For this review, take the finished solid that the model builds, in its own axes (mm). A direction names the side the tool comes from. Coordinates: 2 decimals unless noted, no trailing zeros. Loops run counter-clockwise (first coordinate to the right, second up) from the corner with the lowest first, then second, coordinate; pieces in that order, holes last. Notation, with made-up numbers: M 78.5,-39.75 L 121.5,-39.75 A22 cw 121.5,-12.75 Z; hole C 7,4.5 d7. An arc over 180 degrees is marked long. Put each result on its own line as item: value.
```python
from build123d import *

# Parameters (mm, degrees)
BOSS_EXTRUDE1_DEPTH     = 12
BOSS_EXTRUDE3_DEPTH     = 2
FILLET2_R               = 1
CUT_EXTRUDE7_DEPTH      = 3
CUT_EXTRUDE8_DEPTH      = 1
CUT_EXTRUDE8_DEPTH_BACK = 1


with BuildPart() as part:
    # Sketch1 → Boss-Extrude1 (new body)
    with BuildSketch(Plane.XY):
        with BuildLine():
            Line((3.5, 10), (-3.5, 10))
            ThreePointArc((-3.5, 10), (-5.340169944, 7.795084972), (-6, 5))
            Line((-6, 5), (-6, 0))
            Line((-6, 0), (-7, 0))
            Line((-7, 0), (-7, 1))
            Line((-7, 1), (-7, 5))
            ThreePointArc((-7, 5), (-6.155773268, 8.395374624), (-3.819705149, 11))
            Line((-3.819705149, 11), (3.819705149, 11))
            ThreePointArc((3.819705149, 11), (6.155773268, 8.395374624), (7, 5))
            Line((7, 5), (7, 1))
            Line((7, 1), (7, 0))
            Line((7, 0), (6, 0))
            Line((6, 0), (6, 5))
            ThreePointArc((6, 5), (5.340169944, 7.795084972), (3.5, 10))
        make_face()
    extrude(amount=-BOSS_EXTRUDE1_DEPTH)

    # Sketch4 → Boss-Extrude3 (add)
    with BuildSketch(Plane.XZ):
        with BuildLine():
            Line((-7, 0), (-8.5, 0))
            ThreePointArc((-8.5, 0), (-11.809401077, -3.309401077), (-8.5, -6.618802154))
            Line((-8.5, -6.618802154), (-7, -6.618802154))
            Line((-7, -6.618802154), (-7, 0))
        make_face()
        with BuildLine():
            ThreePointArc((8.5, -6.618802154), (11.809401077, -3.309401077), (8.5, 0))
            Line((8.5, 0), (7, 0))
            Line((7, 0), (7, -6.618802154))
            Line((7, -6.618802154), (8.5, -6.618802154))
        make_face()
    extrude(amount=-BOSS_EXTRUDE3_DEPTH)

    # Fillet2
    fillet2_edges = [part.edges().sort_by_distance(p)[0] for p in [
        (-7, 2, -3.309401077),
        (7, 2, -3.309401077),
    ]]
    fillet(fillet2_edges, radius=FILLET2_R)

    # Sketch5 → Cut-Extrude7 (cut)
    with BuildSketch(Plane(origin=(0, 2, 0), x_dir=(1, 0, 0), z_dir=(0, 1, 0))):
        with BuildLine():
            Line((-7, 4.309401077), (-8, 4.309401077))
            ThreePointArc((-8, 4.309401077), (-9, 3.309401077), (-8, 2.309401077))
            Line((-8, 2.309401077), (-7, 2.309401077))
            Line((-7, 2.309401077), (-3.819705149, 2.309401077))
            Line((-3.819705149, 2.309401077), (-3.819705149, 4.309401077))
            Line((-3.819705149, 4.309401077), (-7, 4.309401077))
        make_face()
        with BuildLine():
            Line((3.819705149, 2.309401077), (7, 2.309401077))
            Line((7, 2.309401077), (8, 2.309401077))
            ThreePointArc((8, 2.309401077), (9, 3.309401077), (8, 4.309401077))
            Line((8, 4.309401077), (7, 4.309401077))
            Line((7, 4.309401077), (3.819705149, 4.309401077))
            Line((3.819705149, 4.309401077), (3.819705149, 2.309401077))
        make_face()
    extrude(amount=-CUT_EXTRUDE7_DEPTH, mode=Mode.SUBTRACT)

    # Sketch6 → Cut-Extrude8 (cut, two sides)
    with BuildSketch(Plane(origin=(0, 2, 0), x_dir=(1, 0, 0), z_dir=(0, 1, 0))) as cut_extrude8_sk:
        Polygon((-8, 5.618802154), (-10, 4.464101615), (-10, 2.154700538), (-8, 1), (-6, 1), (-6, 5.618802154), align=None)
        Polygon((6, 1), (8, 1), (10, 2.154700538), (10, 4.464101615), (8, 5.618802154), (6, 5.618802154), align=None)
    extrude(amount=CUT_EXTRUDE8_DEPTH, mode=Mode.SUBTRACT)
    extrude(cut_extrude8_sk.sketch, amount=-CUT_EXTRUDE8_DEPTH_BACK, mode=Mode.SUBTRACT)


solid = part.part
```
(1) Add section C-C (z = -9). Write out the cut boundary in (x, y).
Determined:
outline: M -7,0 L -6,0 L -6,5 A6.25 cw -3.5,10 L 3.5,10 A6.25 cw 6,5 L 6,0 L 7,0 L 7,5 A7.25 ccw 3.82,11 L -3.82,11 A7.25 ccw -7,5 Z
(2) Add section A-A (y = 4). Write out the cut boundary in (x, z), plus the area to 3 significant figures.
Determined:
outline: M -7,-12 L -6,-12 L -6,0 L -7,0 Z; M 6,-12 L 7,-12 L 7,0 L 6,0 Z
area: 24.0 mm^2
(3) Wall thickness on line 1 along X through (y, z) = (5.25, -4.25) (3 decimals); line 2 along Y through (x, z) = (0.75, -8.25); line 3 along X through (y, z) = (9.25, -9.5): over which ranges is each line inside the solid? List them lowest first. Write a range as [from, to].
Determined:
line 1: x = [-6.996, -5.995], [5.995, 6.996]
line 2: y = [10, 11]
line 3: x = [-5.62, -4.33], [4.33, 5.62]
(4) Add section D-D (y = 1.5). Write out the cut boundary in (x, z), plus the area to 3 significant figures.
Determined:
outline: M -10,-4.46 L -10,-2.15 L -8,-1 L -6,-1 L -6,0 L -8.5,0 A3.31 ccw -8.5,-6.62 L -7,-6.62 L -7,-12 L -6,-12 L -6,-5.62 L -8,-5.62 Z; M 6,-12 L 7,-12 L 7,-6.62 L 8.5,-6.62 A3.31 ccw 8.5,0 L 6,0 L 6,-1 L 8,-1 L 10,-2.15 L 10,-4.46 L 8,-5.62 L 6,-5.62 Z
area: 45.9 mm^2
(5) Draft analysis for pull direction Y (two halves, no side actions). For faces 1 (the flat face through (0, 11, -6)), 2 (the flat face through (6.5, 3, -3.3)), 3 (the flat face through (-9, 1, -4)), 4 (the flat face through (-7, 3, -7)), state which applies: +Y half, -Y half, draft (parallel to the pull), parting line (faces both ways), or undercut.
Determined:
face 1: +Y half
face 2: undercut
face 3: undercut
face 4: draft
(6) Tool access review of faces 5 (the flat face through (-10.4, 2, -3.3)), 6 (the flat face through (7, 2, -1)), 7 (the flat face through (-10, 1.5, -3.3)): name each direction out of +Z, -Z, +X, -X, +Y, -Y from which nothing blocks a thin tool from reaching the whole face with its end or side.
Determined:
face 5: +Z, -Z, -X, +Y
face 6: none
face 7: +Y
(7) For pin 1 (4 mm diameter, centred on y = 3, z = -5.5, fed in from -X); pin 2 (3 mm diameter, centred on x = -10, z = -2, fed in from +Y); pin 3 (1.5 mm diameter, centred on y = 8, z = -9, fed in from +X); pin 4 (2 mm diameter, centred on x = 9.5, z = -10, fed in from -Y), all flat-tipped, find the tip position at first contact; note any pin that passes through.
Determined:
pin 1: stops at x = -11.78
pin 2: stops at y = 2
pin 3: stops at x = 6.64
pin 4: passes through
(8) Add section B-B (z = -5). Write out the cut boundary in (x, y) (3 decimals).
Determined:
outline: M -11.345,0 L -6,0 L -6,1 L -9.072,1 L -9.072,2 L -11.345,2 Z; M -7,3 L -6,3 L -6,5 A6.25 cw -3.5,10 L 3.5,10 A6.25 cw 6,5 L 6,3 L 7,3 L 7,5 A7.25 ccw 3.82,11 L -3.82,11 A7.25 ccw -7,5 Z; M 6,0 L 11.345,0 L 11.345,2 L 9.072,2 L 9.072,1 L 6,1 Z
